Verification items for the finished model (mm, model axes). A direction names the side the tool comes from. Coordinates: 2 decimals unless noted, no trailing zeros. Order: outer loops, then holes, each group sorted by start corner. A loop starts at its lowest first (then second) coordinate and runs counter-clockwise, first axis right, second up. Notation, with made-up numbers: (43.5, 72) - (98.5, 72) arc R19 cw to (98.5, 102) - close; hole circle Ø7 at (-20, 79.25). An arc over 180 degrees is marked (long way). Answer as CSV lines item,"result". Start each with the question number.
1. Mould release check, pull along Z, two halves, no side actions. Record for faces 1 (the flat face through (57.5, 16, 45)), 2 (the flat face through (-1, 5, -60)), 3 (the flat face through (11, 5, -15)), 4 (the flat face through (0, 5, 15.589)): pulls with the +Z half, pulls with the -Z half, needs draft (parallel to the pull), parting line crosses it, or undercut.
2. Set-up check for faces 5 (the flat face through (0, 5, -45.589)), 6 (the flat face through (-20, 0, -1)), 7 (the flat face through (-1, 16, 54)), 8 (the flat face through (-57.5, 16, 45)): record each of +Z, -Z, +X, -X, +Y, -Y from which the full face is reachable in a straight line by a thin tool's end or side.
3. Material ranges on L1, parallel to X at y = 5.25, z = -38.5; L2, parallel to Y at x = -48, z = 18.5; L3, parallel to Z at x = 61.5, y = 5.75, recorded low to high. Write a range as [from, to].
4. Go/stop test with flat-tipped pins: pin 1 (10.5 mm diameter, centred on x = -64.58, z = -45.59, fed in from +Y); pin 2 (9.5 mm diameter, centred on x = 15, y = 17.5, fed in from -Z). Record where each tip stops, or that it passes through.
5. Section check A-A (x = -8). Record the cut outline in (y, z), and give its area (3 significant figures).
6. Section check B-B (z = -31.5). Record the cut outline in (x, y).
7. Section check C-C (y = 2). Record the cut outline in (x, z), and give its area (3 significant figures).
8. Section check D-D (x = 47). Record the cut outline in (y, z), and give its area (3 significant figures).
from build123d import *

# Parameters (mm, degrees)
F_01_BASE_PROFILE_W           = 170
F_01_BASE_PROFILE_H           = 120
F_01_BASE_PROFILE_R           = 4.084295612
F_01_BASE_PROFILE_R_2         = 4.915704388
F_01_BASE_PROFILE_W_2         = 22
F_01_BASE_PROFILE_H_2         = 61.1778291
F_01_BASE_EXTRUDE_DEPTH       = 10
F_02_BOSS_PROFILE_W           = 115
F_02_BOSS_PROFILE_H           = 18
F_02_REINFORCEMENT_BOSS_DEPTH = 22


with BuildPart() as part:
    # 01_Base_Profile → 01_Base_Extrude (new body)
    with BuildSketch(Plane(origin=(0, 0, 0), x_dir=(1, 0, 0), z_dir=(0, 1, 0))):
        Rectangle(F_01_BASE_PROFILE_W, F_01_BASE_PROFILE_H)
        with Locations(Location((-64.584295612, -45.58891455, 0), (0, 0, 270))):
            Circle(F_01_BASE_PROFILE_R, mode=Mode.SUBTRACT)
        with Locations(Location((64.584295612, -45.58891455, 0), (0, 0, 270))):
            Circle(F_01_BASE_PROFILE_R_2, mode=Mode.SUBTRACT)
        with Locations(Location((-64.584295612, 45.58891455, 0), (0, 0, 270))):
            Circle(F_01_BASE_PROFILE_R, mode=Mode.SUBTRACT)
        with Locations(Location((64.584295612, 45.58891455, 0), (0, 0, 270))):
            Circle(F_01_BASE_PROFILE_R_2, mode=Mode.SUBTRACT)
        with Locations((0, 15)):
            Rectangle(F_01_BASE_PROFILE_W_2, F_01_BASE_PROFILE_H_2, mode=Mode.SUBTRACT)
    extrude(amount=F_01_BASE_EXTRUDE_DEPTH)

    # 02_Boss_Profile → 02_Reinforcement_Boss (add)
    with BuildSketch(Plane(origin=(0, 0, 0), x_dir=(1, 0, 0), z_dir=(0, 1, 0))):
        with Locations((0, -45)):
            Rectangle(F_02_BOSS_PROFILE_W, F_02_BOSS_PROFILE_H)
    extrude(amount=F_02_REINFORCEMENT_BOSS_DEPTH)


solid = part.part
Evaluation:
1,face 1,"needs draft"
1,face 2,"pulls with the -Z half"
1,face 3,"undercut"
1,face 4,"undercut"
2,face 5,"+Y, -Y"
2,face 6,"+Z, -Z, +X, -X, -Y"
2,face 7,"+Z, +X, -X, +Y"
2,face 8,"+Z, -Z, -X, +Y"
3,L1,"x = [-85, -11], [11, 85]"
3,L2,"y = [0, 10]"
3,L3,"z = [-60, -49.42], [-41.76, 41.76], [49.42, 60]"
4,pin 1,"stops at y = 10"
4,pin 2,"stops at z = 36"
5,outline,"(0, -60) - (10, -60) - (10, -45.59) - (0, -45.59) - close; (0, 15.59) - (10, 15.59) - (10, 36) - (22, 36) - (22, 54) - (10, 54) - (10, 60) - (0, 60) - close"
5,area,"804 mm²"
6,outline,"(-85, 0) - (-11, 0) - (-11, 10) - (-85, 10) - close; (11, 0) - (85, 0) - (85, 10) - (11, 10) - close"
7,outline,"(-85, -60) - (85, -60) - (85, 60) - (-85, 60) - close; hole circle Ø8.17 at (-64.58, -45.59); hole circle Ø8.17 at (-64.58, 45.59); hole (-11, -45.59) - (11, -45.59) - (11, 15.59) - (-11, 15.59) - close; hole circle Ø9.83 at (64.58, -45.59); hole circle Ø9.83 at (64.58, 45.59)"
7,area,"18,800 mm²"
8,outline,"(0, -60) - (10, -60) - (10, 36) - (22, 36) - (22, 54) - (10, 54) - (10, 60) - (0, 60) - close"
8,area,"1,420 mm²"
